Read the model definition and answer for the solid it produces. Units are mm, in the model's axes. Give positions to 0.01 mm unless a question says otherwise; leave off trailing zeros. Order: outer loops, then holes, each group sorted by start corner. A loop starts at its lowest first (then second) coordinate and runs counter-clockwise, first axis right, second up. Notation, with made-up numbers: (27.25, 2.25) - (61.25, 2.25) arc R17 ccw to (61.25, 35.25) - close; hole circle Ø4 at (-0.75, 34.25). An arc over 180 degrees is marked (long way). One line per item, written item: value. Start each with the question number.
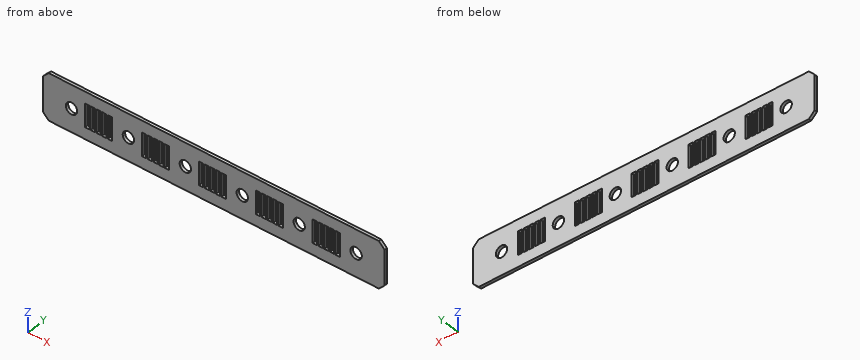
```python
from build123d import *

# Parameters (mm, degrees)
F0_W     = 762
F0_H     = 101.6
F0_R     = 12.7
F1_DEPTH = 6.35
F2_SIZE  = 12.7
F3_W     = 9.525
F3_H     = 50.8
F4_DEPTH = 6.351


with BuildPart() as f1:
    # F0 (on Front) → F1 (new body)
    with BuildSketch(Plane.XZ):
        with Locations((381, 50.8)):
            Rectangle(F0_W, F0_H)
        with Locations((63.5, 50.8)):
            Circle(F0_R, mode=Mode.SUBTRACT)
        with Locations((190.5, 50.8)):
            Circle(F0_R, mode=Mode.SUBTRACT)
        with Locations((317.5, 50.8)):
            Circle(F0_R, mode=Mode.SUBTRACT)
        with Locations((444.5, 50.8)):
            Circle(F0_R, mode=Mode.SUBTRACT)
        with Locations((571.5, 50.8)):
            Circle(F0_R, mode=Mode.SUBTRACT)
        with Locations((698.5, 50.8)):
            Circle(F0_R, mode=Mode.SUBTRACT)
    extrude(amount=F1_DEPTH)

    # F2
    f2_edges = [f1.edges().sort_by_distance(p)[0] for p in [
        (0, -3.175, 101.6),
        (0, -3.175, 0),
        (762, -3.175, 0),
        (762, -3.175, 101.6),
    ]]
    chamfer(f2_edges, length=F2_SIZE)

    # F3 (on face) → F4 (cut, through all)
    with BuildSketch(Plane.XZ.offset(6.35)):
        with Locations((98.4377, 50.8)):
            Rectangle(F3_W, F3_H)
        with Locations((111.1377, 50.8)):
            Rectangle(F3_W, F3_H)
        with Locations((123.8377, 50.8)):
            Rectangle(F3_W, F3_H)
        with Locations((136.5377, 50.8)):
            Rectangle(F3_W, F3_H)
        with Locations((149.2377, 50.8)):
            Rectangle(F3_W, F3_H)
        with Locations((225.4377, 50.8)):
            Rectangle(F3_W, F3_H)
        with Locations((238.1377, 50.8)):
            Rectangle(F3_W, F3_H)
        with Locations((250.8377, 50.8)):
            Rectangle(F3_W, F3_H)
        with Locations((263.5377, 50.8)):
            Rectangle(F3_W, F3_H)
        with Locations((276.2377, 50.8)):
            Rectangle(F3_W, F3_H)
        with Locations((352.4377, 50.8)):
            Rectangle(F3_W, F3_H)
        with Locations((365.1377, 50.8)):
            Rectangle(F3_W, F3_H)
        with Locations((377.8377, 50.8)):
            Rectangle(F3_W, F3_H)
        with Locations((390.5377, 50.8)):
            Rectangle(F3_W, F3_H)
        with Locations((403.2377, 50.8)):
            Rectangle(F3_W, F3_H)
        with Locations((479.4377, 50.8)):
            Rectangle(F3_W, F3_H)
        with Locations((492.1377, 50.8)):
            Rectangle(F3_W, F3_H)
        with Locations((504.8377, 50.8)):
            Rectangle(F3_W, F3_H)
        with Locations((517.5377, 50.8)):
            Rectangle(F3_W, F3_H)
        with Locations((530.2377, 50.8)):
            Rectangle(F3_W, F3_H)
        with Locations((606.4377, 50.8)):
            Rectangle(F3_W, F3_H)
        with Locations((619.1377, 50.8)):
            Rectangle(F3_W, F3_H)
        with Locations((631.8377, 50.8)):
            Rectangle(F3_W, F3_H)
        with Locations((644.5377, 50.8)):
            Rectangle(F3_W, F3_H)
        with Locations((657.2377, 50.8)):
            Rectangle(F3_W, F3_H)
    extrude(amount=-F4_DEPTH, mode=Mode.SUBTRACT)


solid = f1.part
```
1) Find the intervals of material crossed by probe 1 along Z at (x, y) = (444.5, -4.5); probe 2 along Z at (x, y) = (274, -3.75); probe 3 along X at (y, z) = (-3.75, 95.5), in increasing order. Write a range as from..to.
2) Section D-D on x = 69.5 is taken. Write down the section's boundary in (y, z), plus the area to 3 significant figures.
3) Section A-A on x = 190.5 is taken. Write down the section's boundary in (y, z), plus the area to 3 significant figures.
4) Section B-B on y = -4 is taken. Give the number of separate pieces and of enclosed holes in the cut face, plus the area to 3 significant figures.
Solved:
1. probe 1: z = 0..38.1, 63.5..101.6
1. probe 2: z = 0..25.4, 76.2..101.6
1. probe 3: x = 6.6..755.4
2. outline: (-6.35, 0) - (0, 0) - (0, 39.61) - (-6.35, 39.61) - close; (-6.35, 61.99) - (0, 61.99) - (0, 101.6) - (-6.35, 101.6) - close
2. area: 503 mm2
3. outline: (-6.35, 0) - (0, 0) - (0, 38.1) - (-6.35, 38.1) - close; (-6.35, 63.5) - (0, 63.5) - (0, 101.6) - (-6.35, 101.6) - close
3. area: 484 mm2
4. separate pieces: 1
4. enclosed holes: 31
4. area: 62,000 mm2
